```python
from build123d import *

# Parameters (mm, degrees)
CROQUIS1_R              = 2.5
SALIENTE_EXTRUIR1_DEPTH = 10
SALIENTE_EXTRUIR2_DEPTH = 10
CROQUIS10_R             = 2.5
CROQUIS10_R_2           = 12
CROQUIS10_R_3           = 1.5
CORTAR_EXTRUIR1_DEPTH   = 110.854385942


with BuildPart() as part:
    # Croquis1 → Saliente-Extruir1 (new body)
    with BuildSketch(Plane.XY):
        Polygon((-20.5, 39), (-38.5, 39), (-38.5, -39), (38.5, -39), (38.5, 96.757359313), (34.257359313, 101), (-16.257359313, 101), (-20.5, 96.757359313), align=None)
        with Locations((31, 29)):
            Circle(CROQUIS1_R, mode=Mode.SUBTRACT)
        with Locations((31, -29)):
            Circle(CROQUIS1_R, mode=Mode.SUBTRACT)
        with Locations((-31, -29)):
            Circle(CROQUIS1_R, mode=Mode.SUBTRACT)
        with Locations((-31, 29)):
            Circle(CROQUIS1_R, mode=Mode.SUBTRACT)
    extrude(amount=SALIENTE_EXTRUIR1_DEPTH)

    # Croquis9 → Saliente-Extruir2 (add, through all)
    with BuildSketch(Plane.XY.offset(10)):
        Polygon((-38.5, 35.464466094), (-38.5, 18.393398282), (-34.964466094, 39), align=None)
        Polygon((-42.035533906, 21.928932188), (-38.5, 18.393398282), (-38.5, 35.464466094), (-42.035533906, 31.928932188), align=None)
        Polygon((34.964466094, 39), (38.5, 18.393398282), (38.5, 35.464466094), align=None)
        Polygon((38.5, 35.464466094), (38.5, 18.393398282), (42.035533906, 21.928932188), (42.035533906, 31.928932188), align=None)
        Polygon((38.5, -21.928932188), (38.5, -30.464466094), (38.5, -39), (42.035533906, -35.464466094), (42.035533906, -25.464466094), align=None)
        Polygon((29.964466094, -39), (21.428932188, -39), (24.964466094, -42.535533906), (34.964466094, -42.535533906), (38.5, -39), align=None)
        Polygon((38.5, -30.464466094), (29.964466094, -39), (38.5, -39), align=None)
        Polygon((-38.5, -39), (-38.5, -30.464466094), (-38.5, -21.928932188), (-42.035533906, -25.464466094), (-42.035533906, -35.464466094), align=None)
        Polygon((-38.5, -39), (-29.964466094, -39), (-38.5, -30.464466094), align=None)
        Polygon((-24.964466094, -42.535533906), (-21.428932188, -39), (-29.964466094, -39), (-38.5, -39), (-34.964466094, -42.535533906), align=None)
        Polygon((-20.5, 42.168004936), (-23.668004936, 39), (-20.5, 39), align=None)
    extrude(amount=-SALIENTE_EXTRUIR2_DEPTH)

    # Croquis10 → Cortar-Extruir1 (cut, through all)
    with BuildSketch(Plane.XY.offset(10)):
        Polygon((-38.5, 39), (-38.5, 35.464466094), (-34.964466094, 39), align=None)
        with Locations((25, 72)):
            Circle(CROQUIS10_R)
        with Locations((25, 91)):
            Circle(CROQUIS10_R)
        with Locations((0.5, 37)):
            Circle(CROQUIS10_R_2)
        with Locations((-14.5, 52)):
            Circle(CROQUIS10_R_3)
        with Locations((15.5, 52)):
            Circle(CROQUIS10_R_3)
        with Locations((15.5, 22)):
            Circle(CROQUIS10_R_3)
        with Locations((-14.5, 22)):
            Circle(CROQUIS10_R_3)
    extrude(amount=-CORTAR_EXTRUIR1_DEPTH, mode=Mode.SUBTRACT)


solid = part.part
```
Model file for the job. Use its own axes, mm. A direction names the side the tool comes from. Coordinates: 2 decimals unless noted, no trailing zeros. Write each loop counter-clockwise with the first axis right and the second up, starting at its lowest first coordinate (ties: lowest second). Pieces come first, ordered by that corner, then holes. Notation, with made-up numbers: (60, 26) - (99, 26) arc R31 ccw to (99, 53) - close; hole circle Ø4 at (81.25, 89). An arc over 180 degrees is marked (long way). Use a Markdown table: item, result. Add a question column.
Item 1: 3-axis set-ups, long thin cutter, end or side, ignore diameter. For faces 5 (the face through (-30, -42.536, 5)), 6 (the face through (23.17, -40.74, 5.07)), 7 (the face through (-38.5, -1, 5)): which of +Z, -Z, +X, -X, +Y, -Y reach the whole face in a straight line?
Item 2: Band-saw the part on B-B, the plane y = -29. Write the cut outline in (x, z), and give its area (3 significant figures).
Item 3: Band-saw the part on C-C, the plane x = 0.5. Write the cut outline in (y, z).
Item 4: Drill centre lines: line 1 along Y through (x, z) = (15.5, 5.75); line 2 along Y through (x, z) = (25, 3.5); line 3 along X through (y, z) = (59, 4). Where is each one in solid material? Low to high.
Item 5: Two-plate mould, pull along X, no slides. Class faces 1 (the face through (30.67, -26.52, 4.93)), 2 (the face through (42.036, 27, 5)), 3 (the face through (-1, 14, 10)), 4 (the face through (-38.5, -39, 5.1)): pulls with the +X half, pulls with the -X half, needs draft (parallel to the pull), parting line crosses it, or undercut.
Item 6: Band-saw the part on A-A, the plane x = 31. Write the cut outline in (y, z), and give its area (3 significant figures).
Item 7: Band-saw the part on D-D, the plane y = 91. Write the cut outline in (x, z).
Item 8: Drop flat-ended pins along their axis: pin 1 (3 mm diameter, centred on y = 60.5, z = 3.5, fed in from +X); pin 2 (4 mm diameter, centred on x = 21.5, z = 3.5, fed in from -Y); pin 3 (3 mm diameter, centred on y = 83, z = 6.5, fed in from -X). Give the stop position or say it passes through.
A:
| question | item | result |
|---|---|---|
| 1 | face 5 | +Z, -Z, +X, -X, -Y |
| 1 | face 6 | +Z, -Z, -Y |
| 1 | face 7 | +Z, -Z, -X |
| 2 | outline | (-42.04, 0) - (-33.5, 0) - (-33.5, 10) - (-42.04, 10) - close; (-28.5, 0) - (28.5, 0) - (28.5, 10) - (-28.5, 10) - close; (33.5, 0) - (42.04, 0) - (42.04, 10) - (33.5, 10) - close |
| 2 | area | 741 mm² |
| 3 | outline | (-39, 0) - (25, 0) - (25, 10) - (-39, 10) - close; (49, 0) - (101, 0) - (101, 10) - (49, 10) - close |
| 4 | line 1 | y = -39 to 20.5, 23.5 to 50.5, 53.5 to 101 |
| 4 | line 2 | y = -42.54 to 69.5, 74.5 to 88.5, 93.5 to 101 |
| 4 | line 3 | x = -20.5 to 38.5 |
| 5 | face 1 | undercut |
| 5 | face 2 | pulls with the +X half |
| 5 | face 3 | needs draft |
| 5 | face 4 | pulls with the -X half |
| 6 | outline | (-42.54, 0) - (-31.5, 0) - (-31.5, 10) - (-42.54, 10) - close; (-26.5, 0) - (26.5, 0) - (26.5, 10) - (-26.5, 10) - close; (31.5, 0) - (101, 0) - (101, 10) - (31.5, 10) - close |
| 6 | area | 1,340 mm² |
| 7 | outline | (-20.5, 0) - (22.5, 0) - (22.5, 10) - (-20.5, 10) - close; (27.5, 0) - (38.5, 0) - (38.5, 10) - (27.5, 10) - close |
| 8 | pin 1 | stops at x = 38.5 |
| 8 | pin 2 | stops at y = -41.07 |
| 8 | pin 3 | stops at x = -20.5 |
